```python
from build123d import *

# Parameters (mm, degrees)
F0_R     = 11.2
F1_DEPTH = 7
F2_R     = 1.5
F3_DEPTH = 7


# Not quite as in the source:
# - a feature names something its author has since deleted; it is built from what else it names


with BuildPart() as f1:
    # F0 (on Top) → F1 (new body)
    with BuildSketch(Plane.XY):
        with BuildLine():
            ThreePointArc((22.3972222345, -0.1780444605), (11.6219084102, 6.8053952105), (11.1419447663, 19.6368196267))
            ThreePointArc((11.1419447663, 19.6368196267), (-0.0899760733, 39.914441113), (-11.0444200915, 19.4855856595))
            ThreePointArc((-11.0444200915, 19.4855856595), (-11.7045993402, 6.6621703185), (-22.5769570295, -0.1692025982))
            ThreePointArc((-22.5769570295, -0.1692025982), (-34.5219319451, -20.0351421217), (-11.352802143, -19.3075411991))
            ThreePointArc((-11.352802143, -19.3075411991), (0.08269093, -13.467565529), (11.4350122631, -19.4676170286))
            ThreePointArc((11.4350122631, -19.4676170286), (34.6119080183, -19.8792989913), (22.3972222345, -0.1780444605))
        make_face()
        with Locations((-23.1356502259, -13.3573738858)):
            Circle(F0_R, mode=Mode.SUBTRACT)
        with Locations((23.1356502259, -13.3573738858)):
            Circle(F0_R, mode=Mode.SUBTRACT)
        Circle(F0_R, mode=Mode.SUBTRACT)
        with Locations((0, 26.7147477716)):
            Circle(F0_R, mode=Mode.SUBTRACT)
    extrude(amount=F1_DEPTH)

    # F2 (call 1 of 2: OpenCascade refuses the feature's edges together)
    f2_edges = [f1.edges().sort_by_distance(p)[0] for p in [
        (-34.521932, -20.035142, 7),
        (-11.704599, 6.66217, 7),
        (34.611908, -19.879299, 7),
        (-0.089976, 39.914441, 7),
        (0.082691, -13.467566, 7),
        (11.621908, 6.805395, 7),
    ]]
    fillet(f2_edges, radius=F2_R)

    # F2#2 (call 2 of 2)
    f2_2_edges = [f1.edges().sort_by_distance(p)[0] for p in [
        (34.611908, -19.879299, 0),
        (0.082691, -13.467566, 0),
        (-34.521932, -20.035142, 0),
        (-0.089976, 39.914441, 0),
        (11.621908, 6.805395, 0),
        (-11.704599, 6.66217, 0),
    ]]
    fillet(f2_2_edges, radius=F2_R)

    # F0 (on Top) → F3 (join)
    with BuildSketch(Plane.XY):
        with BuildLine():
            ThreePointArc((22.3972222345, -0.1780444605), (11.6219084102, 6.8053952105), (11.1419447663, 19.6368196267))
            ThreePointArc((11.1419447663, 19.6368196267), (-0.0899760733, 39.914441113), (-11.0444200915, 19.4855856595))
            ThreePointArc((-11.0444200915, 19.4855856595), (-11.7045993402, 6.6621703185), (-22.5769570295, -0.1692025982))
            ThreePointArc((-22.5769570295, -0.1692025982), (-34.5219319451, -20.0351421217), (-11.352802143, -19.3075411991))
            ThreePointArc((-11.352802143, -19.3075411991), (0.08269093, -13.467565529), (11.4350122631, -19.4676170286))
            ThreePointArc((11.4350122631, -19.4676170286), (34.6119080183, -19.8792989913), (22.3972222345, -0.1780444605))
        make_face()
        with Locations((-23.1356502259, -13.3573738858)):
            Circle(F0_R, mode=Mode.SUBTRACT)
        with Locations((23.1356502259, -13.3573738858)):
            Circle(F0_R, mode=Mode.SUBTRACT)
        Circle(F0_R, mode=Mode.SUBTRACT)
        with Locations((0, 26.7147477716)):
            Circle(F0_R, mode=Mode.SUBTRACT)
    extrude(amount=F3_DEPTH)


solid = f1.part
```
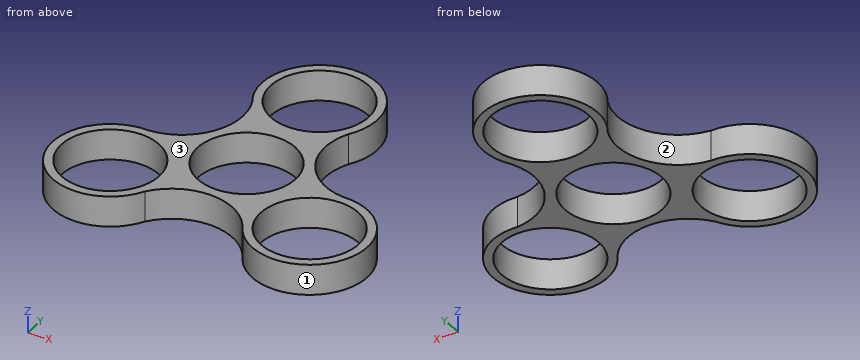
CAD build for the part. Positions are in the model's coordinates, mm. Face numbers are marked on the shaded views. Give positions to 0.01 mm unless a question says otherwise; leave off trailing zeros. Loops run counter-clockwise (first coordinate to the right, second up) from the corner with the lowest first, then second, coordinate; pieces in that order, holes last. Notation, with made-up numbers: (30.5, -28) - (73.5, -28) arc R18 cw to (73.5, -20) - close; hole circle Ø11 at (79.25, 79.25). An arc over 180 degrees is marked (long way). Put each result on its own line as item: value.
Q1. Probe line 1 along Y through (x, z) = (0, 3.5); line 2 along X through (y, z) = (-19, 1.25); line 3 along X through (y, z) = (-22.5, 5.5) (1 decimal). List the from-to ranges inside material, lowest first.
Filled in:
line 1: y = -13.47 to -11.2, 11.2 to 15.51, 37.91 to 39.91
line 2: x = -35.07 to -32.81, -13.46 to -11.13, 11.1 to 13.46, 32.81 to 35.07
line 3: x = -32.7 to -29.6, -16.7 to -13.6, 13.6 to 16.7, 29.6 to 32.7
Q2. Flat gauge pins, fed straight in: pin 1 (1 mm diameter, centred on x = -3.5, z = 4.5, fed in from -Y); pin 2 (3 mm diameter, centred on x = -5, z = 2.5, fed in from +Y). Where does each tip first touch, or does it go through?
Filled in:
pin 1: stops at y = -14.05
pin 2: stops at y = 39.44
Q3. Slice it at A-A (x = 0). Give the cut face in (y, z).
Filled in:
outline: (-13.47, 0) - (-11.2, 0) - (-11.2, 7) - (-13.47, 7) - close; (11.2, 0) - (15.51, 0) - (15.51, 7) - (11.2, 7) - close; (37.91, 0) - (39.91, 0) - (39.91, 7) - (37.91, 7) - close
Q4. Slice it at D-D (x = 18). Give the cut face in (y, z), plus the area to 3 significant figures.
Filled in:
outline: (-25.52, 0) - (-23.31, 0) - (-23.31, 7) - (-25.52, 7) - close; (-3.4, 0) - (0.99, 0) - (0.99, 7) - (-3.4, 7) - close
area: 46.2 mm²
Q5. Mould opens along Y. For the marked faces 1, 2 and 3 say: pulls with the +Y half, pulls with the -Y half, needs draft (parallel to the pull), parting line crosses it, or undercut.
Filled in:
face 1: parting line crosses it
face 2: undercut
face 3: needs draft
Q6. Slice it at C-C (y = 33). Give the cut face in (x, z), plus the area to 3 significant figures.
Filled in:
outline: (-11.61, 0) - (-9.27, 0) - (-9.27, 7) - (-11.61, 7) - close; (9.27, 0) - (11.61, 0) - (11.61, 7) - (9.27, 7) - close
area: 32.7 mm²
Q7. Slice it at B-B (y = -5.5). Give the cut face in (x, z).
Filled in:
outline: (-33.74, 0) - (-31.12, 0) - (-31.12, 7) - (-33.74, 7) - close; (-15.15, 0) - (-9.76, 0) - (-9.76, 7) - (-15.15, 7) - close; (9.76, 0) - (15.15, 0) - (15.15, 7) - (9.76, 7) - close; (31.12, 0) - (33.74, 0) - (33.74, 7) - (31.12, 7) - close
